Could you check a few things on this model? Use its own coordinates, in mm. Face numbers are marked on the shaded views. A direction names the side the tool comes from. Coordinates: 2 decimals unless noted, no trailing zeros. Loops run counter-clockwise (first coordinate to the right, second up) from the corner with the lowest first, then second, coordinate; pieces in that order, holes last. Notation, with made-up numbers: (-27, -10) - (17, -10) arc R23 cw to (17, 18) - close; hole circle Ø2 at (18, -18.75). An arc over 180 degrees is marked (long way). Use CSV: the item, a comma, the result in double quotes.
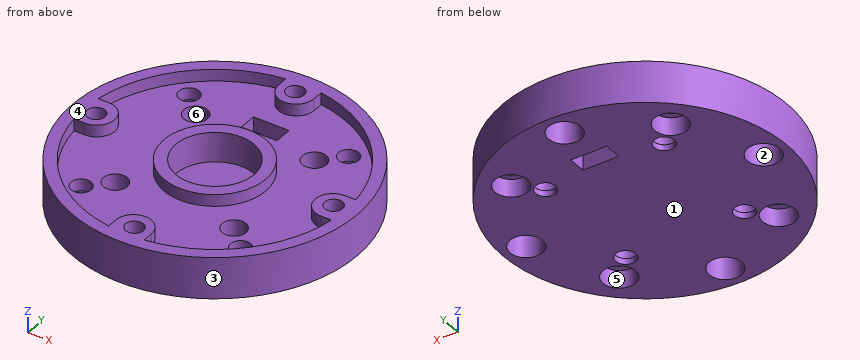
from build123d import *

# Parameters (mm, degrees)
REVOLVE_ONTO_SKETCH002_ROLL_ANGLE = 90
ARRAY_COUNT                       = 4
PAD_DEPTH                         = 2
POLARPATTERN_COUNT                = 4
SKETCH005_R                       = 1.7
POCKET_DEPTH                      = 141.485431
POLARPATTERN001_COUNT             = 4
SKETCH006_R                       = 1.7
POCKET001_DEPTH                   = 5.001
SKETCH007_R                       = 2
POCKET002_DEPTH                   = 4
SKETCH008_R                       = 2.75
POCKET003_DEPTH                   = 3
SKETCH009_W                       = 6
SKETCH009_H                       = 3
POCKET004_DEPTH                   = 5.001


with BuildPart() as array:
    # Sketch002 as drawn → Revolve (revolve)
    with BuildSketch(Plane.XY):
        Polygon((17.25, -1), (17.25, 4), (18.5, 4), (18.5, 8), (20, 8), (20, -1), align=None)
    revolve(axis=Axis((20, 8, 0), (0, -1, 0)))


with BuildPart() as array_1:
    # Revolve onto Sketch002 roll: moved
    add(array.part.rotate(Axis((0, 0, 0), (1, 0, 0)), REVOLVE_ONTO_SKETCH002_ROLL_ANGLE))


with BuildPart() as array_2:
    # Revolve onto Sketch002 placement: moved
    add(array_1.part)

    # Array: Array ×4 about axis
    array_axis = Axis((0, 0, 0), (0, 0, 1))


with BuildPart() as array_3:
    add(array_2.part)
    for i in range(1, ARRAY_COUNT):
        add(array_2.part.rotate(array_axis, i * 360 / ARRAY_COUNT))


with BuildPart() as pocket004:
    # Sketch → Revolution (revolve)
    with BuildSketch(Plane.XZ):
        Polygon((0, 0), (24, 0), (24, 7), (22, 7), (22, 5), (8.6, 5), (8.6, 7), (6.6, 7), (6.6, 2), (0, 2), align=None)
    revolve(axis=Axis((0, 0, 0), (0, 0, 1)))

    # Sketch004 → Pad (new body)
    with BuildSketch(Plane(origin=(0, 0, 7), x_dir=(-1, 0, 0), z_dir=(0, 0, 1))):
        with BuildLine():
            Line((-22, 3.164727), (-20, 3.164727))
            ThreePointArc((-20, -2.835273), (-17, 0.164727), (-20, 3.164727))
            Line((-20, -2.835273), (-22, -2.835273))
            Line((-22, -2.835273), (-22, 3.164727))
        make_face()
    pad = extrude(amount=-PAD_DEPTH)

    # PolarPattern: Pad ×4 about axis
    polarpattern_axis = Axis((0, 0, 7), (0, 0, 1))
    for i in range(1, POLARPATTERN_COUNT):
        add(pad.rotate(polarpattern_axis, i * 360 / POLARPATTERN_COUNT))

    # Cut: cut Array
    add(array_3.part, mode=Mode.SUBTRACT)

    # Sketch005 → Pocket (cut, through all)
    with BuildSketch(Plane.XY.offset(5)):
        with Locations((-13.435029, 13.435029)):
            Circle(SKETCH005_R)
    pocket = extrude(amount=-POCKET_DEPTH, mode=Mode.SUBTRACT)

    # PolarPattern001: Pocket ×4 about axis
    polarpattern001_axis = Axis((0, 0, 5), (0, 0, 1))
    for i in range(1, POLARPATTERN001_COUNT):
        add(pocket.rotate(polarpattern001_axis, i * 360 / POLARPATTERN001_COUNT), mode=Mode.SUBTRACT)

    # Sketch006 → Pocket001 (cut, through all)
    with BuildSketch(Plane.XY.offset(5)):
        with Locations((10, 10)):
            Circle(SKETCH006_R)
        with Locations((-10, 10)):
            Circle(SKETCH006_R)
        with Locations((-10, -10)):
            Circle(SKETCH006_R)
        with Locations((10, -10)):
            Circle(SKETCH006_R)
    extrude(amount=-POCKET001_DEPTH, mode=Mode.SUBTRACT)

    # Sketch007 → Pocket002 (cut)
    with BuildSketch(Plane.XY.offset(5)):
        with Locations((-10, -10)):
            Circle(SKETCH007_R)
        with Locations((10, -10)):
            Circle(SKETCH007_R)
        with Locations((10, 10)):
            Circle(SKETCH007_R)
        with Locations((-10, 10)):
            Circle(SKETCH007_R)
    extrude(amount=-POCKET002_DEPTH, mode=Mode.SUBTRACT)

    # Sketch008 → Pocket003 (cut)
    with BuildSketch(Plane(origin=(0, 0, 0), x_dir=(1, 0, 0), z_dir=(0, 0, -1))):
        with Locations((-13.435029, 13.435029)):
            Circle(SKETCH008_R)
        with Locations((-13.435029, -13.435029)):
            Circle(SKETCH008_R)
        with Locations((13.435029, -13.435029)):
            Circle(SKETCH008_R)
        with Locations((13.435029, 13.435029)):
            Circle(SKETCH008_R)
    extrude(amount=-POCKET003_DEPTH, mode=Mode.SUBTRACT)

    # Sketch009 → Pocket004 (cut, through all)
    with BuildSketch(Plane.XY.offset(5)):
        with Locations((0, 12.5)):
            Rectangle(SKETCH009_W, SKETCH009_H)
    extrude(amount=-POCKET004_DEPTH, mode=Mode.SUBTRACT)


solid = pocket004.part
(1) Suppose I cut it at A-A (z = 6). Write out the boundary of the cut face in (x, y), plus the area to 3 significant figures.
Computed:
outline,"circle Ø48 at (0, 0); circle Ø17.2 at (0, 0); hole (-21.82, -2.84) arc R22 ccw to (-3.16, -21.77) - (-3.16, -20) arc R3 cw to (2.84, -20) - (2.84, -21.82) arc R22 ccw to (21.77, -3.16) - (20, -3.16) arc R3 cw to (20, 2.84) - (21.82, 2.84) arc R22 ccw to (3.16, 21.77) - (3.16, 20) arc R3 cw to (-2.84, 20) - (-2.84, 21.82) arc R22 ccw to (-21.77, 3.16) - (-20, 3.16) arc R3 cw to (-20, -2.84) - close; hole circle Ø3 at (-20, 0); hole circle Ø13.2 at (0, 0); hole circle Ø3 at (0, -20); hole circle Ø3 at (0, 20); hole circle Ø3 at (20, 0)"
area,"459 mm²"
(2) Which directions (+Z, -Z, +X, -X, +Y, -Y) give clear straight access to the entire face, cutting with the end or side of a thin tool? Please do the marked faces 4, 5 and 6.
Computed:
face 4,"+Z, +X, -X, +Y, -Y"
face 5,"-Z"
face 6,"+Z"
(3) Suppose I cut it at B-B (y = 10). Write out the boundary of the cut face in (x, z).
Computed:
outline,"(-21.82, 0) - (-11.7, 0) - (-11.7, 1) - (-12, 1) - (-12, 5) - (-19.6, 5) - (-19.6, 7) - (-21.82, 7) - close; (-8.3, 0) - (8.3, 0) - (8.3, 1) - (8, 1) - (8, 5) - (-8, 5) - (-8, 1) - (-8.3, 1) - close; (11.7, 0) - (21.82, 0) - (21.82, 7) - (19.6, 7) - (19.6, 5) - (12, 5) - (12, 1) - (11.7, 1) - close"
(4) Please list where these lines run through material, in increasing order: line 1 (Y direction, x = 10, z = 3.5); line 2 (X direction, y = 1, z = 1); line 3 (X direction, y = -14.5, z = 2.75).
Computed:
line 1,"y = -21.82 to -12, -8 to 8, 12 to 21.82"
line 2,"x = -23.98 to -22.56, -17.44 to 17.44, 22.56 to 23.98"
line 3,"x = -19.12 to -15.97, -10.9 to 10.9, 15.97 to 19.12"
(5) Thinking about a two-plate mould opening in Y: for the marked faces 1, 2 and 3, which applies, +Y half, -Y half, draft (parallel to the pull), parting line (faces both ways), or undercut?
Computed:
face 1,"draft"
face 2,"undercut"
face 3,"parting line"
(6) Suppose I cut it at D-D (x = -5.5). Write out the boundary of the cut face in (y, z), plus the area to 3 significant figures.
Computed:
outline,"(-23.36, 0) - (23.36, 0) - (23.36, 7) - (21.3, 7) - (21.3, 5) - (6.61, 5) - (6.61, 7) - (3.65, 7) - (3.65, 2) - (-3.65, 2) - (-3.65, 7) - (-6.61, 7) - (-6.61, 5) - (-21.3, 5) - (-21.3, 7) - (-23.36, 7) - close"
area,"232 mm²"
(7) Will these pins go through, and if not, where does the flat tip stop? pin 1 (3 mm diameter, centred on x = 15.5, z = 5, fed in from +Y); pin 2 (4 mm diameter, centred on y = 12.5, z = 1, fed in from +X); pin 3 (1.9 mm diameter, centred on x = -21, z = 6.5, fed in from +Y); pin 4 (2.5 mm diameter, centred on x = 20, y = 0, fed in from -Z).
Computed:
pin 1,"stops at y = 19.49"
pin 2,"stops at x = 21.58"
pin 3,"stops at y = 13.19"
pin 4,"passes through"
